Geometry check sheet. Reference: the model listing, model coordinates, mm. A direction names the side the tool comes from. Round coordinates to 2 decimals unless told otherwise and drop trailing zeros. Order: outer loops, then holes, each group sorted by start corner. A loop starts at its lowest first (then second) coordinate and runs counter-clockwise, first axis right, second up. Notation, with made-up numbers: (76, 40.5) - (135, 40.5) arc R11 cw to (135, 51.5) - close; hole circle Ø8 at (-7, 12.5). An arc over 180 degrees is marked (long way). Return JSON: item names as keys, results as strings. Group by question number.
Q1. Sectioned sample at A-A, the plane z = 0. Record the cut outline in (x, y), then the cut area to 3 significant figures.
Q2. Sectioned sample at B-B, the plane z = -8. Record the cut outline in (x, y), then the cut area to 3 significant figures.
Q3. Sectioned sample at C-C, the plane x = -4. Record the cut outline in (y, z), then the cut area to 3 significant figures.
Q4. Gauge pin test, flat ends, axial feed: pin 1 Ø2.5 at (x, z) = (-8, 0) entering from +Y (1 decimal); pin 2 Ø5 at (x, z) = (8, 0) entering from +Y; pin 3 Ø2 at (x, y) = (-4, 4) entering from +Z; pin 4 Ø2 at (y, z) = (9, -5.5) entering from +X. Record the tip position at first contact, or that the pin passes through.
Q5. Tool access check on faces 1 (the cylindrical face through (-0.35, 1, -9.56)), 2 (the cylindrical face through (1.08, 7.08, -4.88)). Record the directions out of +Z, -Z, +X, -X, +Y, -Y that give a thin tool (end or side, any length) a straight path to the whole face; none if there is none.
Q6. Material ranges on line 1 along Z through (x, y) = (0, 6.5); line 2 along Z through (x, y) = (-8, 1.05); line 3 along Y through (x, z) = (6.5, -5.5), recorded low to high.
Q7. Sectioned sample at D-D, the plane y = 10. Record the cut outline in (x, z).
Q8. Draft check along X on faces 3 (the flat face through (0.2, 2.014, -5.4)), 4 (the cylindrical face through (-0.35, 1, 6.44)), 5 (the cylindrical face through (-11.923, 1.028, 3.755)). Enter one of: pulls with the +X half, pulls with the -X half, needs draft (parallel to the pull), parting line crosses it, or undercut.
```python
from build123d import *

# Parameters (mm, degrees)
SKETCH_2_R          = 1.6
CUT_EXTRUDE_1_DEPTH = 10


with BuildPart() as part:
    # 草图1 → 旋转1 (revolve)
    with BuildSketch(Plane.XY):
        Polygon((-2.5, 0.013967073), (-12.5, 0.013967073), (-12.5, 2.013967073), (-5, 2.013967073), (-5, 12.013967073), (-2.5, 12.013967073), align=None)
    revolve(axis=Axis((0, 0, 0), (0, 1, 0)))

    # 草图2 → 切除-拉伸1 (cut)
    with BuildSketch(Plane.XZ.offset(-0.013967073)):
        with Locations((-8, 0)):
            Circle(SKETCH_2_R)
        with Locations((0, 8)):
            Circle(SKETCH_2_R)
        with Locations((8, 0)):
            Circle(SKETCH_2_R)
        with Locations((0, -8)):
            Circle(SKETCH_2_R)
    extrude(amount=-CUT_EXTRUDE_1_DEPTH, mode=Mode.SUBTRACT)


solid = part.part
```
Reply:
{
 "1": {"outline": "(-12.5, 0.01) - (-9.6, 0.01) - (-9.6, 2.01) - (-12.5, 2.01) - close; (-6.4, 0.01) - (-2.5, 0.01) - (-2.5, 12.01) - (-5, 12.01) - (-5, 2.01) - (-6.4, 2.01) - close; (2.5, 0.01) - (6.4, 0.01) - (6.4, 2.01) - (5, 2.01) - (5, 12.01) - (2.5, 12.01) - close; (9.6, 0.01) - (12.5, 0.01) - (12.5, 2.01) - (9.6, 2.01) - close", "area": "77.2 mm^2"},
 "2": {"outline": "(-9.6, 0.01) - (-1.6, 0.01) - (-1.6, 2.01) - (-9.6, 2.01) - close; (1.6, 0.01) - (9.6, 0.01) - (9.6, 2.01) - (1.6, 2.01) - close", "area": "32.0 mm^2"},
 "3": {"outline": "(0.01, -11.84) - (2.01, -11.84) - (2.01, -3) - (12.01, -3) - (12.01, 3) - (2.01, 3) - (2.01, 11.84) - (0.01, 11.84) - close", "area": "107 mm^2"},
 "4": {"pin 1": "through", "pin 2": "y = 2.01", "pin 3": "z = 4", "pin 4": "x = 2.18"},
 "5": {"face 1": "+Y, -Y", "face 2": "+Y"},
 "6": {"line 1": "-5 to -2.5, 2.5 to 5", "line 2": "-9.6 to -1.6, 1.6 to 9.6", "line 3": "0.01 to 2.01"},
 "7": {"outline": "circle Ø10 at (0, 0); hole circle Ø5 at (0, 0)"},
 "8": {"face 3": "needs draft", "face 4": "undercut", "face 5": "parting line crosses it"}
}
